Build history of the part. All positions in model axes, mm. Face numbers are marked on the shaded views. A direction names the side the tool comes from. Coordinates: 2 decimals unless noted, no trailing zeros. Write each loop counter-clockwise with the first axis right and the second up, starting at its lowest first coordinate (ties: lowest second). Pieces come first, ordered by that corner, then holes. Notation, with made-up numbers: (-29.5, 78) -> (15.5, 78) arc R15 ccw to (15.5, 96) -> close; hole circle Ø6 at (43, -34.5). An arc over 180 degrees is marked (long way). Write each question's results on one line, items separated by ' | '. Start each with the question number.
Q1. Drill centre lines: line 1 (X direction, y = -40, z = 75); line 2 (Z direction, x = -15.5, y = -15.5); line 3 (X direction, y = 21.5, z = 106.5). Where is each one in solid material? Low to high.
Q2. Saw through at A-A on y = 24.5. Give the cut face in (x, z).
Q3. Drop flat-ended pins along their axis: pin 1 Ø10 at (x, z) = (0.5, 71) entering from +Y; pin 2 Ø1 at (x, y) = (-68.5, -40.5) entering from -Z. Give the stop position or say it passes through.
Q4. Saw through at D-D on x = -56. Give the cut face in (y, z).
Q5. Saw through at B-B on y = -2.5. Give the cut face in (x, z), and give its area (3 significant figures).
Q6. Saw through at C-C on z = 9. Give the cut face in (x, y), and give its area (3 significant figures).
Q7. Tool access for the marked faces 1 and 2: list every direction of +Z, -Z, +X, -X, +Y, -Y with a clear straight run to the whole face (end or side of a thin tool).
Q8. Two-plate mould, pull along X, no slides. Class the marked faces 3, 4, 5 and 6: released by +X, released by -X, zero draft, split by the parting line, or undercut.
from build123d import *

# Parameters (mm, degrees)
F0_W      = 269.0858095884
F0_H      = 136.0893808305
F1_DEPTH  = 127
F2_R      = 42.6246558772
F3_DEPTH  = 127.001
F5_DEPTH  = 25.4
F7_DEPTH  = 25.4
F8_R      = 12.8692359505
F9_DEPTH  = 136.0903808305
F10_R     = 11.8876823155
F11_DEPTH = 136.0903808305


with BuildPart() as f1:
    # F0 (on Top) → F1 (new body)
    with BuildSketch(Plane.XY):
        with Locations((-20.9878012538, -17.8948733956)):
            Rectangle(F0_W, F0_H)
    extrude(amount=F1_DEPTH)

    # F2 (on face) → F3 (cut, through all)
    with BuildSketch(Plane.XY.offset(127)):
        with Locations((-20.9878012538, 50.1498170197)):
            Circle(F2_R)
    extrude(amount=-F3_DEPTH, mode=Mode.SUBTRACT)

    # F4 (on face) → F5 (join)
    with BuildSketch(Plane(origin=(0, 0, 0), x_dir=(1, 0, 0), z_dir=(0, 0, -1))):
        with BuildLine():
            Line((21.6368546234, -50.1498170197), (40.624178946, -50.1498170197))
            ThreePointArc((40.624178946, -50.1498170197), (-20.9878012538, 12.1844288341), (-82.5997814536, -50.1498170197))
            Line((-82.5997814536, -50.1498170197), (-63.612457131, -50.1498170197))
            ThreePointArc((-63.612457131, -50.1498170197), (-20.9878012538, -7.6825284563), (21.6368546234, -50.1498170197))
        make_face()
    extrude(amount=F5_DEPTH)

    # F6 (on face) → F7 (join)
    with BuildSketch(Plane.XY.offset(127)):
        with BuildLine():
            ThreePointArc((21.6368546234, 50.1498170197), (-20.9878012538, 7.6304695536), (-63.612457131, 50.1498170197))
            Line((-63.612457131, 50.1498170197), (-82.5997814536, 50.1498170197))
            ThreePointArc((-82.5997814536, 50.1498170197), (-20.9878012538, -13.3016428499), (40.624178946, 50.1498170197))
            Line((40.624178946, 50.1498170197), (21.6368546234, 50.1498170197))
        make_face()
    extrude(amount=F7_DEPTH)

    # F8 (on face) → F9 (cut, through all)
    with BuildSketch(Plane(origin=(0, 50.1498170197, 0), x_dir=(-1, 0, 0), z_dir=(0, 1, 0))):
        with Locations((98.3830988407, 63.9618188143)):
            Circle(F8_R)
    extrude(amount=-F9_DEPTH, mode=Mode.SUBTRACT)

    # F10 (on face) → F11 (cut, through all)
    with BuildSketch(Plane.XZ.offset(85.9395638108)):
        with Locations((60.9713494778, 65.8634230494)):
            Circle(F10_R)
    extrude(amount=-F11_DEPTH, mode=Mode.SUBTRACT)


solid = f1.part
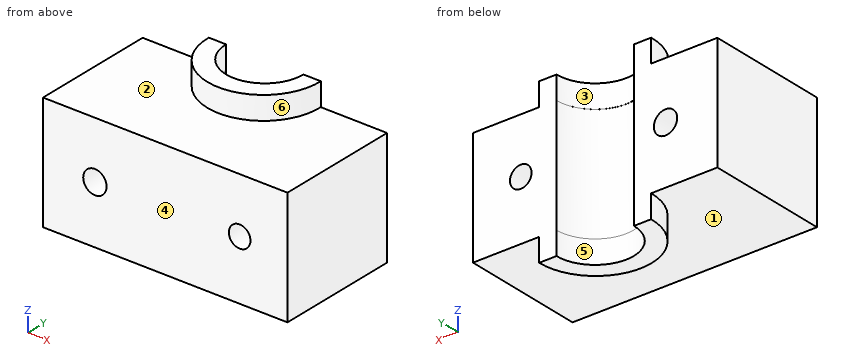
Returned:
1) line 1: x = -155.53 to -105, -91.77 to 53.37, 68.58 to 113.56 | line 2: z = 0 to 127 | line 3: x = -155.53 to -52.55, 10.57 to 113.56
2) outline: (-155.53, 0) -> (-77.33, 0) -> (-77.33, -25.4) -> (-54.91, -25.4) -> (-54.91, 0) -> (-55.03, 0) -> (-55.03, 127) -> (-54.95, 127) -> (-54.95, 152.4) -> (-77.83, 152.4) -> (-77.83, 127) -> (-155.53, 127) -> close; (12.94, -25.4) -> (35.36, -25.4) -> (35.36, 0) -> (113.56, 0) -> (113.56, 127) -> (35.86, 127) -> (35.86, 152.4) -> (12.98, 152.4) -> (12.98, 127) -> (13.06, 127) -> (13.06, 0) -> (12.94, 0) -> close; hole circle Ø25.74 at (-98.38, 63.96); hole circle Ø23.78 at (60.97, 65.86)
3) pin 1: stops at y = 16.75 | pin 2: stops at z = 0
4) outline: (-85.94, 0) -> (-1.27, 0) -> (-1.27, -25.4) -> (26, -25.4) -> (26, 0) -> (25.84, 0) -> (25.84, 127) -> (25.94, 127) -> (25.94, 152.4) -> (-2.39, 152.4) -> (-2.39, 127) -> (-85.94, 127) -> close
5) outline: (-155.53, 0) -> (-54.15, 0) -> (-54.15, -25.4) -> (12.17, -25.4) -> (12.17, 0) -> (113.56, 0) -> (113.56, 127) -> (13.87, 127) -> (13.87, 152.4) -> (-55.84, 152.4) -> (-55.84, 127) -> (-155.53, 127) -> close; hole circle Ø25.74 at (-98.38, 63.96); hole circle Ø23.78 at (60.97, 65.86) | area: 36,700 mm2
6) outline: (-155.53, -85.94) -> (113.56, -85.94) -> (113.56, 50.15) -> (21.64, 50.15) arc R42.62 cw to (-63.61, 50.15) -> (-155.53, 50.15) -> close | area: 33,800 mm2
7) face 1: -Z, -Y | face 2: +Z, -Y
8) face 3: undercut | face 4: zero draft | face 5: undercut | face 6: split by the parting line
